Geometry: final body of the model. Coordinates: model frame, mm. A direction names the side the tool comes from. Round coordinates to 2 decimals unless told otherwise and drop trailing zeros. Loops run counter-clockwise (first coordinate to the right, second up) from the corner with the lowest first, then second, coordinate; pieces in that order, holes last. Notation, with made-up numbers: M 9,-10.5 L 13,-10.5 A24 ccw 13,11.5 Z; hole C 26,45.25 d3. An arc over 180 degrees is marked long. Answer as a JSON object with one key per item and string values.
from build123d import *

# Parameters (mm, degrees)
POLARPATTERN_COUNT = 4


with BuildPart() as part:
    # Sketch371 → Revolution001 (revolve)
    with BuildSketch(Plane.XZ):
        Polygon((-109.5, 0.8), (-97.3, 0.8), (-97.3, -6), (-98.5, -6), (-98.5, 0), (-109.5, 0), align=None)
    revolve(axis=Axis((0, 0, 0), (0, 0, 1)))

    # Sketch372 (on DatumPlane) → Revolution002 (revolve)
    with BuildSketch(Plane(origin=(104, 0, 0), x_dir=(1, 0, 0), z_dir=(0, -1, 0))):
        Polygon((2.35, -6), (2.35, -0.85), (3.2, 0), (0.925, 0), (0.925, -6), align=None)
    revolution002 = revolve(axis=Axis((104, 0, 0), (0, 0, 1)))

    # PolarPattern: Revolution002 ×4 about axis
    polarpattern_axis = Axis((0, 0, 0), (0, 0, 1))
    for i in range(1, POLARPATTERN_COUNT):
        add(revolution002.rotate(polarpattern_axis, i * 360 / POLARPATTERN_COUNT))


with BuildPart() as part_1:
    # Body022078 placement: moved
    add(part.part.moved(Location((0, 0, -144.5))))


solid = part_1.part
1) Section query A-A (z = -148). Count the separate pieces of the cut face and the enclosed holes in it, and give its area (3 significant figures).
Results:
{"separate pieces": "5", "enclosed holes": "5", "area": "797 mm2"}
2) Reachability of faces 1 (the cylindrical face through (-0.103, 101.652, -147.889)), 2 (the cylindrical face through (23.737, 106.896, -144.094)) from +Z, -Z, +X, -X, +Y, -Y: full face, straight path, thin tool, end or side. Return the list, or none.
Results:
{"face 1": "-Z", "face 2": "+Z, -Z"}
3) Section query C-C (y = -13). Return the cut outline in (x, z).
Results:
{"outline": "M -108.73,-144.5 L -97.64,-144.5 L -97.64,-150.5 L -96.43,-150.5 L -96.43,-143.7 L -108.73,-143.7 Z; M 96.43,-150.5 L 97.64,-150.5 L 97.64,-144.5 L 108.73,-144.5 L 108.73,-143.7 L 96.43,-143.7 Z"}
4) Pin query (flat end, axial travel): P1, Ø4, axis at x = -34, z = -147.5, coming from the +Y side; P2, Ø1, axis at y = 6.5, z = -149.5, coming from the -X side; P3, Ø1.7, axis at x = 0, y = 104, coming from the -Z side. Return the tip coordinate at first contact, or that it passes through.
Results:
{"P1": "y = 93.16", "P2": "x = -98.32", "P3": "z = -144.5"}
5) Pull-direction query (Y, two-part tool) for faces 3 (the cylindrical face through (-92.807, -29.226, -147.148)), 4 (the cylindrical face through (101.652, 0.103, -147.889)), 5 (the flat face through (1, -98, -143.7)); classes: +Y half, -Y half, draft (parallel to the pull), parting line (faces both ways), or undercut.
Results:
{"face 3": "undercut", "face 4": "parting line", "face 5": "draft"}
6) Section query B-B (x = -76). Return the cut outline in (y, z).
Results:
{"outline": "M -78.83,-144.5 L -62.66,-144.5 L -62.66,-150.5 L -60.76,-150.5 L -60.76,-143.7 L -78.83,-143.7 Z; M 60.76,-150.5 L 62.66,-150.5 L 62.66,-144.5 L 78.83,-144.5 L 78.83,-143.7 L 60.76,-143.7 Z"}
7) Ray query, line 1 (X direction, y = 1.5, z = -146); line 2 (X direction, y = 104, z = -146) (3 decimals); line 3 (X direction, y = 65, z = -145.5). Return the intervals inside material, ascending.
Results:
{"line 1": "-105.81 to -102.19, -98.49 to -97.29, 97.29 to 98.49, 102.19 to 105.81", "line 2": "-2.35 to -0.925, 0.925 to 2.35", "line 3": "-74.01 to -72.4, 72.4 to 74.01"}
